Check sheet for the modelled part. Datum: model origin and axes. Units: mm. A direction names the side the tool comes from. Give positions to 0.01 mm unless a question says otherwise; leave off trailing zeros. Loops run counter-clockwise (first coordinate to the right, second up) from the corner with the lowest first, then second, coordinate; pieces in that order, holes last. Notation, with made-up numbers: M -10.5,55 L 4.5,55 A14 cw 4.5,81 Z; hole C -10,-28 d9. An arc over 180 degrees is marked long. Use one line per item in the form item = value.
Autodesk Inventor part; units mm, degrees
ref_plane "YZ Plane" through (0, 0, 0) normal (1, 0, 0) x (0, 1, 0)
ref_plane "XZ Plane" through (0, 0, 0) normal (0, 1, 0) x (-1, 0, 0)
ref_plane "XY Plane" through (0, 0, 0) normal (0, 0, 1) x (1, 0, 0)
sketch "Esquisse1" plane through (0, 0, 0) normal (1, 0, 0) x (0, 1, 0)
  line L0 (0, 0) -> (-200, 0)
  line L1 (-200, 0) -> (-200, -20)
  line L2 (-200, -20) -> (-20, -290)
  line L3 (-20, -290) -> (0, -290)
  line L4 (0, -290) -> (0, 0)
  dimension "d0" = 200
  dimension "d1" = 20
  dimension "d2" = 20
  dimension "d3" = 290
extrude "Extrusion1" add sketch "Esquisse1" along normal blind 18.55
sketch "Esquisse2" plane through (18.55, 0, 0) normal (1, 0, 0) x (0, 0, -1)
  line L0 (0, 0) -> (0, -200)
  line L1 (0, -50) -> (-18.55, -50)
  line L2 (-18.55, -50) -> (-18.55, -150)
  line L3 (-18.55, -150) -> (0, -150)
  line L4 (0, -150) -> (0, -50)
  line L5 (290, 0) -> (0, 0)
  point P0 (0, -150)
  dimension "d6" = 18.55
  dimension "d7" = 50
  dimension "d8" = 100
extrude "Extrusion2" add sketch "Esquisse2" against normal blind 18.55
sketch "Esquisse3" plane through (18.55, 0, 0) normal (1, 0, 0) x (0, 0, -1)
  circle A0 centre (-1.1314, -48.8686) radius 1.6
  line L0 (-1.1314, -48.8686) -> (0, -50) construction
  line L1 (0, -50) -> (-18.55, -50)
  circle A1 centre (-1.1314, -151.1314) radius 1.6
  point P0 (0, 0)
  point P1 (0, -150)
  dimension "d12" = 3.2
  dimension "d11" = 45
extrude "Extrusion3" cut sketch "Esquisse3" against normal blind 18.55
properties part number "Bracket"
1) Depth check by flat-ended pin: pin 1 Ø9.5 at (x, y) = (12, -184) entering from +Z; pin 2 Ø10 at (x, y) = (2.5, -125) entering from -Z; pin 3 Ø8 at (x, z) = (8, 12.5) entering from +Y. Enter the tip coordinate at first touch or a pass-through.
Evaluation:
pin_1 = 0
pin_2 = -140
pin_3 = -50
2) Section check C-C (z = -101.5). Record the cut outline in (x, y), then the cut area to 3 significant figures.
Evaluation:
outline = M 0,-145.67 L 18.55,-145.67 L 18.55,0 L 0,0 Z
area = 2,700 mm^2
3) Section check B-B (y = -92). Record the cut outline in (x, z).
Evaluation:
outline = M 0,-182 L 18.55,-182 L 18.55,18.55 L 0,18.55 Z
4) Scan lines: line 1 (Z direction, x = 1, y = -12.5); line 2 (Y direction, x = 16.75, z = -255.5); line 3 (Y direction, x = 3, z = -113.5). Record each from-to range of solid material in increasing order.
Evaluation:
line_1 = -290 to 0
line_2 = -43 to 0
line_3 = -137.67 to 0
5) Section check A-A (x = 4). Record the cut outline in (y, z).
Evaluation:
outline = M -200,-20 L -20,-290 L 0,-290 L 0,0 L -47.74,0 A1.6 cw -50,2.26 L -50,18.55 L -150,18.55 L -150,2.26 A1.6 cw -152.26,0 L -200,0 Z
6) Set-up check for faces 1 (the face through (9, -176, 0)), 2 (the face through (9, -24, 0)), 3 (the face through (9.15, -111.26, -153.11)): record each of +Z, -Z, +X, -X, +Y, -Y from which the full face is reachable in a straight line by a thin tool's end or side.
Evaluation:
face_1 = +Z, +X, -X, -Y
face_2 = +Z, +X, -X, +Y
face_3 = -Z, +X, -X, -Y
